```python
from build123d import *

# Parameters (mm, degrees)
BOSS_EXTRUDE1_DEPTH      = 76.2
BOSS_EXTRUDE1_DEPTH_BACK = 76.2
CUT_EXTRUDE1_DEPTH       = 82.319677815


with BuildPart() as part:
    # Sketch4 → Boss-Extrude1 (new, two sides: drawn at the far end of the back side and taken through both)
    with BuildSketch(Plane(origin=(0, 0, 0), x_dir=(0, 0, -1), z_dir=(1, 0, 0)).offset(-BOSS_EXTRUDE1_DEPTH_BACK)):
        with BuildLine():
            Line((12.7, -11.43), (12.7, 11.43))
            ThreePointArc((12.7, 11.43), (12.328025612, 12.328025612), (11.43, 12.7))
            Line((11.43, 12.7), (-11.43, 12.7))
            ThreePointArc((-11.43, 12.7), (-12.328025612, 12.328025612), (-12.7, 11.43))
            Line((-12.7, 11.43), (-12.7, -11.43))
            ThreePointArc((-12.7, -11.43), (-12.328025612, -12.328025612), (-11.43, -12.7))
            Line((-11.43, -12.7), (11.43, -12.7))
            ThreePointArc((11.43, -12.7), (12.328025612, -12.328025612), (12.7, -11.43))
        make_face()
        with BuildLine():
            Line((11.049, 9.9441), (11.049, -9.9441))
            ThreePointArc((11.049, -9.9441), (10.725382283, -10.725382283), (9.9441, -11.049))
            Line((9.9441, -11.049), (-9.9441, -11.049))
            ThreePointArc((-9.9441, -11.049), (-10.725382283, -10.725382283), (-11.049, -9.9441))
            Line((-11.049, -9.9441), (-11.049, 9.9441))
            ThreePointArc((-11.049, 9.9441), (-10.725382283, 10.725382283), (-9.9441, 11.049))
            Line((-9.9441, 11.049), (9.9441, 11.049))
            ThreePointArc((9.9441, 11.049), (10.725382283, 10.725382283), (11.049, 9.9441))
        make_face(mode=Mode.SUBTRACT)
    extrude(amount=BOSS_EXTRUDE1_DEPTH + BOSS_EXTRUDE1_DEPTH_BACK)

    # Sketch5 → Cut-Extrude1 (cut, through all)
    with BuildSketch(Plane.XY.offset(12.7)):
        Polygon((76.2, -12.7), (76.2, 12.7), (70.568955569, 12.7), align=None)
        Polygon((-76.2, -12.7), (-76.2, 12.7), (-70.568955569, -12.7), align=None)
    extrude(amount=-CUT_EXTRUDE1_DEPTH, mode=Mode.SUBTRACT)


solid = part.part
```
CAD build for the part. Positions are in the model's coordinates, mm. A direction names the side the tool comes from. Round coordinates to 2 decimals unless told otherwise and drop trailing zeros. Order: outer loops, then holes, each group sorted by start corner. A loop starts at its lowest first (then second) coordinate and runs counter-clockwise, first axis right, second up. Notation, with made-up numbers: (28, 11.25) -> (60, 11.25) arc R34 ccw to (60, 50.25) -> close; hole circle Ø10 at (18.25, 23.5). An arc over 180 degrees is marked (long way). Write item = value, one per line.
(1) Cut at B-B (z = -2.5). Write the cut outline in (x, y).
Answers follow:
outline = (-76.2, 12.7) -> (-75.83, 11.05) -> (70.93, 11.05) -> (70.57, 12.7) -> close; (-70.93, -11.05) -> (-70.57, -12.7) -> (76.2, -12.7) -> (75.83, -11.05) -> close
(2) 3-axis set-ups, long thin cutter, end or side, ignore diameter. For faces 5 (the flat face through (-3, 11.049, 0)), 6 (the flat face through (-1, 0, 12.7)): which of +Z, -Z, +X, -X, +Y, -Y reach the whole face in a straight line?
Answers follow:
face_5 = +X, -X
face_6 = +Z, +X, -X, +Y, -Y
(3) Drill centre lines: L1, parallel to Y at x = 47, z = 4.25; L2, parallel to Z at x = -12.5, y = 10.75. Where is each one in solid material? Low to high.
Answers follow:
L1 = -12.7 to -11.05, 11.05 to 12.7
L2 = -12.7 to -10.7, 10.7 to 12.7
(4) Cut at C-C (y = 2). Write the cut outline in (x, z).
Answers follow:
outline = (-73.83, -12.7) -> (72.94, -12.7) -> (72.94, -11.05) -> (-73.83, -11.05) -> close; (-73.83, 11.05) -> (72.94, 11.05) -> (72.94, 12.7) -> (-73.83, 12.7) -> close
(5) Pull direction Y, two halves, no side cores. Call faces 1 (the flat face through (-1, 0, -12.7)), 2 (the flat face through (-4, 12.7, 0)), 3 (the flat face through (2, -12.7, 0)), 4 (the flat face through (-1, 0, 11.049)): +Y half, -Y half, draft (parallel to the pull), parting line (faces both ways), or undercut.
Answers follow:
face_1 = draft
face_2 = +Y half
face_3 = -Y half
face_4 = undercut
(6) Cut at A-A (x = -52.5). Write the cut outline in (y, z).
Answers follow:
outline = (-12.7, -11.43) arc R1.27 ccw to (-11.43, -12.7) -> (11.43, -12.7) arc R1.27 ccw to (12.7, -11.43) -> (12.7, 11.43) arc R1.27 ccw to (11.43, 12.7) -> (-11.43, 12.7) arc R1.27 ccw to (-12.7, 11.43) -> close; hole (-11.05, -9.94) arc R1.1 ccw to (-9.94, -11.05) -> (9.94, -11.05) arc R1.1 ccw to (11.05, -9.94) -> (11.05, 9.94) arc R1.1 ccw to (9.94, 11.05) -> (-9.94, 11.05) arc R1.1 ccw to (-11.05, 9.94) -> close
